Can you work these out from the model? Positions are in its coordinate system, mm. A direction names the side the tool comes from. Give positions to 0.01 mm unless a question says otherwise; leave off trailing zeros. Order: outer loops, then holes, each group sorted by start corner. A loop starts at its lowest first (then second) coordinate and runs counter-clockwise, first axis right, second up. Notation, with made-up numbers: M 80.5,8 L 128.5,8 A15 ccw 128.5,31 Z; hole C 85,70.25 d3. An arc over 180 degrees is marked long. Use one line per item in the form item = value. Start each with the question number.
1. I want a section at D-D, the plane z = -10. List the corners of the cut face in (x, y) for me, and give its area (3 significant figures).
2. For faces 4 (the face through (0, 16, -9.5)), 5 (the face through (-9, 2, -5)), which set-ups out of +Z, -Z, +X, -X, +Y, -Y let a thin tool reach every point of the face, with its end or its side?
3. I want a section at A-A, the plane y = 12.5. List the corners of the cut face in (x, z) for me, and give its area (3 significant figures).
4. We'd pull the mould along X, two halves only. Please class faces 1 (the face through (9, 2, -5)), 2 (the face through (-0.1, 9.5, -12.5)), 3 (the face through (-2.027, 14.359, -10.979)): +X half, -X half, draft (parallel to the pull), parting line (faces both ways), or undercut.
5. Will these pins go through, and if not, where does the flat tip stop? P1, Ø1, axis at x = 1.5, z = -4, coming from the +Y side; P2, Ø3, axis at x = 6.5, y = 22, coming from the +Z side.
6. I want a section at B-B, the plane z = 0. List the corners of the cut face in (x, y) for me.
7. I need wall thicknesses on L1, parallel to X at y = 2, z = 0; L2, parallel to Y at x = 0, z = -11; L3, parallel to Z at x = -5.75, y = 19. Which ranges of each line are inside material? Lowest first, please.
8. I want a section at C-C, the plane x = 0. List the corners of the cut face in (y, z) for me.
```python
from build123d import *

# Parameters (mm, degrees)
SKETCH_1_W          = 18
SKETCH_1_H          = 25
SKETCH_1_R          = 2.75
EXTRUDE_1_DEPTH     = 3
SKETCH_2_W          = 18
SKETCH_2_H          = 3
EXTRUDE_2_DEPTH     = 22
SKETCH_3_R          = 2.75
CUT_EXTRUDE_1_DEPTH = 22


with BuildPart() as part:
    # 草图1 → 凸台-拉伸1 (new body)
    with BuildSketch(Plane(origin=(0, 0, 0), x_dir=(1, 0, 0), z_dir=(0, 1, 0))):
        Rectangle(SKETCH_1_W, SKETCH_1_H)
        with Locations(Location((0, 0, 0), (0, 0, 270))):
            Circle(SKETCH_1_R, mode=Mode.SUBTRACT)
    extrude(amount=EXTRUDE_1_DEPTH)

    # 草图2 → 凸台-拉伸2 (add)
    with BuildSketch(Plane(origin=(0, 3, 0), x_dir=(1, 0, 0), z_dir=(0, 1, 0))):
        with Locations((0, 11)):
            Rectangle(SKETCH_2_W, SKETCH_2_H)
    extrude(amount=EXTRUDE_2_DEPTH)

    # 草图3 → 切除-拉伸1 (cut)
    with BuildSketch(Plane.XY.offset(-9.5)):
        with Locations((0, 12.5)):
            Circle(SKETCH_3_R)
    extrude(amount=-CUT_EXTRUDE_1_DEPTH, mode=Mode.SUBTRACT)


solid = part.part
```
Check result:
q1.outline = M -9,0 L 9,0 L 9,25 L -9,25 Z; hole C 0,12.5 d5.5
q1.area = 426 mm2
q2.face_4 = +Z, +X, -X, +Y
q2.face_5 = +Z, -Z, -X, +Y, -Y
q3.outline = M -9,-12.5 L -2.75,-12.5 L -2.75,-9.5 L -9,-9.5 Z; M 2.75,-12.5 L 9,-12.5 L 9,-9.5 L 2.75,-9.5 Z
q3.area = 37.5 mm2
q4.face_1 = +X half
q4.face_2 = draft
q4.face_3 = undercut
q5.P1 = 3
q5.P2 = -9.5
q6.outline = M -9,0 L -2.75,0 L -2.75,3 L -9,3 Z; M 2.75,0 L 9,0 L 9,3 L 2.75,3 Z
q7.L1 = -9 to -2.75, 2.75 to 9
q7.L2 = 0 to 9.75, 15.25 to 25
q7.L3 = -12.5 to -9.5
q8.outline = M 0,-12.5 L 9.75,-12.5 L 9.75,-9.5 L 3,-9.5 L 3,-2.75 L 0,-2.75 Z; M 0,2.75 L 3,2.75 L 3,12.5 L 0,12.5 Z; M 15.25,-12.5 L 25,-12.5 L 25,-9.5 L 15.25,-9.5 Z
